from build123d import *

# Parameters (mm, degrees)
BOSS_EXTRUDE1_DEPTH = 25.4
FILLET1_R           = 25.4
SKETCH2_R           = 2.794
CUT_EXTRUDE1_DEPTH  = 77.2
CUT_EXTRUDE2_START  = -6.35
SKETCH3_R           = 4.064
CUT_EXTRUDE2_DEPTH  = 70.850000033
FILLET2_R           = 1.5875


with BuildPart() as part:
    # Sketch1 → Boss-Extrude1 (new body)
    with BuildSketch(Plane(origin=(0, 0, 0), x_dir=(0, 0, -1), z_dir=(1, 0, 0))):
        Polygon((0, 0), (0, 50.8), (6.35, 50.8), (6.35, 11.43), (50.8, 11.43), (50.8, 0), align=None)
    extrude(amount=BOSS_EXTRUDE1_DEPTH)

    # Fillet1
    fillet1_edges = [part.edges().sort_by_distance(p)[0] for p in [
        (12.7, 11.43, -6.35),
    ]]
    fillet(fillet1_edges, radius=FILLET1_R)

    # Sketch2 → Cut-Extrude1 (cut, through all)
    with BuildSketch(Plane.XY):
        with Locations((6.35, 41.275)):
            Circle(SKETCH2_R)
        with Locations((6.35, 15.875)):
            Circle(SKETCH2_R)
        with Locations(Location((19.05, 41.275, 0), (0, 0, 270))):
            Circle(SKETCH2_R)
        with Locations((19.05, 15.875)):
            Circle(SKETCH2_R)
    extrude(amount=-CUT_EXTRUDE1_DEPTH, mode=Mode.SUBTRACT)

    # Sketch3 → Cut-Extrude2 (cut, through all)
    with BuildSketch(Plane.XY.offset(CUT_EXTRUDE2_START)):
        with Locations((6.35, 15.875)):
            Circle(SKETCH3_R)
        with Locations((19.05, 15.875)):
            Circle(SKETCH3_R)
    extrude(amount=-CUT_EXTRUDE2_DEPTH, mode=Mode.SUBTRACT)

    # Fillet2
    fillet2_edges = [part.edges().sort_by_distance(p)[0] for p in [
        (12.7, 11.43, -50.8),
        (12.7, 0, -50.8),
        (25.4, 11.43, -41.275),
        (0, 43.815, -6.35),
        (25.4, 43.815, -6.35),
        (25.4, 50.8, -3.175),
        (0, 18.869487758, -13.789487758),
        (25.4, 18.869487758, -13.789487758),
        (25.4, 0, -25.4),
        (0, 50.8, -3.175),
        (0, 11.43, -41.275),
        (0, 5.715, -50.8),
        (0, 0, -25.4),
        (25.4, 5.715, -50.8),
    ]]
    fillet(fillet2_edges, radius=FILLET2_R)


solid = part.part
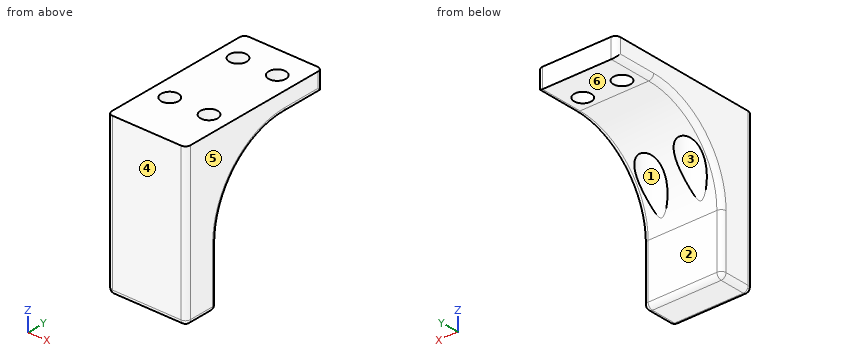
Geometry check sheet. Reference: the model listing, model coordinates, mm. Face numbers are marked on the shaded views. A direction names the side the tool comes from. Round coordinates to 2 decimals unless told otherwise and drop trailing zeros. One line per question, with ' | ' between items. Start each with the question number.
(1) Sectioned sample at A-A on x = 17.5. Count the separate pieces of the cut face and the enclosed holes in it, and give its area (3 significant figures).
(2) Access from +Z, -Z, +X, -X, +Y, -Y to the whole of each face (thin tool, end or side, straight path). Record for the marked faces 5 and 6.
(3) Depth check by flat-ended pin: pin 1 Ø4 at (y, z) = (13, -25.5) entering from +X; pin 2 Ø5 at (x, y) = (6.35, 41.275) entering from -Z; pin 3 Ø8.5 at (x, z) = (18.5, -41.5) entering from +Y; pin 4 Ø7.5 at (x, y) = (6.35, 15.875) entering from -Z. Enter the tip coordinate at first touch or a pass-through.
(4) Thickness scan on L1, parallel to Y at x = 6.25, z = -6; L2, parallel to Y at x = 7.5, z = -2.5; L3, parallel to Z at x = 23, y = 49.5. Record the ranges inside material, lowest first. Write a range as [from, to].
(5) Release check for a two-part mould opening along Y. For the marked faces 1, 2, 3 and 4 record: released by +Y, released by -Y, zero draft, split by the parting line, or undercut.
Conclusion:
1) separate pieces: 3 | enclosed holes: 0 | area: 821 mm2
2) face 5: +Z, -Z, +X, +Y, -Y | face 6: -Z, +X, -X, +Y
3) pin 1: stops at x = 25.36 | pin 2: passes through | pin 3: stops at y = 11.43 | pin 4: stops at z = -6.35
4) L1: y = [0, 13.08], [18.67, 38.48], [44.07, 50.8] | L2: y = [0, 13.33], [18.42, 38.73], [43.82, 50.8] | L3: z = [-6.35, 0]
5) face 1: undercut | face 2: released by +Y | face 3: undercut | face 4: released by -Y
